Work out the finished part from the listing and answer in its coordinate system (mm). Coordinates: 2 decimals unless noted, no trailing zeros. Loops run counter-clockwise (first coordinate to the right, second up) from the corner with the lowest first, then second, coordinate; pieces in that order, holes last. Notation, with made-up numbers: M 20,66.25 L 48,66.25 A33 ccw 48,94.25 Z; hole C -15,40 d4. An arc over 180 degrees is marked long. Write each question's results on one line, items separated by ' | '.
Autodesk Inventor part; units mm, degrees
ref_plane "YZ Plane" through (0, 0, 0) normal (1, 0, 0) x (0, 1, 0)
ref_plane "XZ Plane" through (0, 0, 0) normal (0, 1, 0) x (-1, 0, 0)
ref_plane "XY Plane" through (0, 0, 0) normal (0, 0, 1) x (1, 0, 0)
sketch "Sketch1" plane through (0, 0, 0) normal (0, 0, 1) x (1, 0, 0)
  point P0 (0, 0)
sketch "Sketch2" plane through (0, 0, 0) normal (0, 0, 1) x (1, 0, 0)
  line L0 (0, 0) -> (150, 0)
  line L1 (150, 0) -> (150, 50)
  line L2 (150, 50) -> (0, 50)
  line L3 (0, 50) -> (0, 0)
  dimension "d0" = 150
  dimension "d1" = 50
extrude "Extrusion1" add sketch "Sketch2" along normal blind 5
sketch "Sketch3" plane through (0, 0, 5) normal (0, 0, 1) x (1, 0, 0)
  line L0 (0, 0) -> (0, 25)
  line L1 (0, 50) -> (0, 0)
  arc A0 (20.6375, 23.8125) -> (0, 25) centre (0, -154.9228) ccw
  dimension "d4" = 25
sketch "Sketch4" plane through (0, 0, 5) normal (0, 0, 1) x (1, 0, 0)
  point P0 (0, 0)
sketch "Sketch5" plane through (0, 0, 5) normal (0, 0, 1) x (1, 0, 0)
  line L0 (0, 0) -> (150, 0)
  line L1 (150, 0) -> (150, 25)
  line L2 (150, 0) -> (150, 50)
  dimension "d5" = 25
sketch "Sketch6" plane through (0, 0, 5) normal (0, 0, 1) x (1, 0, 0)
  line L0 (150, 0) -> (150, 50)
  line L1 (150, 25) -> (90, 25)
  line L2 (90, 25) -> (60, 25)
  line L3 (60, 25) -> (0, 25)
  line L4 (0, 25) -> (75, 25)
  circle A0 centre (75, 25) radius 15
  point P0 (0, 0)
  dimension "d6" = 60
  dimension "d7" = 30
  dimension "d8" = 60
  dimension "d9" = 75
  dimension "d10" = 30
extrude "Extrusion2" cut sketch "Sketch6" against normal through all
properties part number "kj"
1) Given pin 1 Ø24 at (x, y) = (75, 25) entering from +Z, flat-ended and moving along its own axis, determine where the tip first touches the part or whether it passes through.
Check result:
pin 1: through
2) Find section A-A, the plane y = 25. Give the vertices of the cut face in (x, z).
Check result:
outline: M 0,0 L 60,0 L 60,5 L 0,5 Z; M 90,0 L 150,0 L 150,5 L 90,5 Z
3) For a pull along X with two mould halves and no side action, classify faces 1 (the face through (63, 16, 3)), 2 (the face through (150, 25, 2)), 3 (the face through (74, 9, 0)) as released by +X, released by -X, zero draft, split by the parting line, or undercut.
Check result:
face 1: undercut | face 2: released by +X | face 3: zero draft
4) Straight lines are drawn through the part: probe 1 along Y at (x, z) = (75, 1.05); probe 2 along X at (y, z) = (25, 1.85); probe 3 along Y at (x, z) = (79.5, 3.45). For each, find the intervals that lie inside material, in ascending order. Write a range as [from, to].
Check result:
probe 1: [0, 10], [40, 50] | probe 2: [0, 60], [90, 150] | probe 3: [0, 10.69], [39.31, 50]
5) Find section B-B, the plane x = 75. Give the vertices of the cut face in (y, z), and give its area (3 significant figures).
Check result:
outline: M 0,0 L 10,0 L 10,5 L 0,5 Z; M 40,0 L 50,0 L 50,5 L 40,5 Z | area: 100 mm^2
6) Find section C-C, the plane z = 1.35. Give the vertices of the cut face in (x, y).
Check result:
outline: M 0,0 L 150,0 L 150,50 L 0,50 Z; hole C 75,25 d30
